from build123d import *

# Parameters (mm, degrees)
SKETCH_1_W               = 25
SKETCH_1_H               = 15
EXTRUDE_1_DEPTH          = 22
FILLET_4_R               = 2
CUT_EXTRUDE_3_DEPTH      = 27.391286441
CUT_EXTRUDE_3_DEPTH_BACK = 27.391286441
CUT_EXTRUDE_4_DEPTH      = 27.391286441
CUT_EXTRUDE_4_DEPTH_BACK = 27.391286441
SKETCH_3_R               = 1
CUT_EXTRUDE_5_DEPTH      = 30.41513216
CUT_EXTRUDE_5_DEPTH_BACK = 30.41513216
SKETCH_4_W               = 13
SKETCH_4_H               = 15
SKETCH_5_W               = 15
SKETCH_5_H               = 7
CUT_EXTRUDE_6_DEPTH      = 35.135758377
FILLET_5_R               = 1


with BuildPart() as part:
    # 草图1 → 凸台-拉伸1 (new body)
    with BuildSketch(Plane.XY):
        Rectangle(SKETCH_1_W, SKETCH_1_H)
    extrude(amount=EXTRUDE_1_DEPTH)

    # 圆角4
    fillet_4_edges = [part.edges().sort_by_distance(p)[0] for p in [
        (12.5, -7.5, 11),
        (-12.5, -7.5, 11),
        (-12.5, 7.5, 11),
        (12.5, 7.5, 11),
    ]]
    fillet(fillet_4_edges, radius=FILLET_4_R)

    # 草图2 → 切除-拉伸3 (cut, two sides: drawn at the far end of the back side and taken through both)
    with BuildSketch(Plane.XY.offset(22).offset(-CUT_EXTRUDE_3_DEPTH_BACK)):
        with BuildLine():
            Line((-10.5, 0.062323454), (-10.5, -0.062323454))
            ThreePointArc((-10.5, -0.062323454), (-10.125727394, -0.842365266), (-9.283069542, -1.038510514))
            Line((-9.283069542, -1.038510514), (-9.002613999, -0.97618706))
            ThreePointArc((-9.002613999, -0.97618706), (-8.219544457, 0), (-9.002613999, 0.97618706))
            Line((-9.002613999, 0.97618706), (-9.283069542, 1.038510514))
            ThreePointArc((-9.283069542, 1.038510514), (-10.125727394, 0.842365266), (-10.5, 0.062323454))
        make_face()
        with BuildLine():
            Line((0.216930458, 1.072600597), (8.997386001, 3.02381294))
            ThreePointArc((8.997386001, 3.02381294), (9.774484481, 4.109116772), (8.780455543, 5))
            Line((8.780455543, 5), (-8.780455543, 5))
            ThreePointArc((-8.780455543, 5), (-9.774484481, 4.109116772), (-8.997386001, 3.02381294))
            Line((-8.997386001, 3.02381294), (-0.216930458, 1.072600597))
            ThreePointArc((-0.216930458, 1.072600597), (0, 1.048787657), (0.216930458, 1.072600597))
        make_face()
        with BuildLine():
            Line((9.283069542, 1.038510514), (9.002613999, 0.97618706))
            ThreePointArc((9.002613999, 0.97618706), (8.219544457, 0), (9.002613999, -0.97618706))
            Line((9.002613999, -0.97618706), (9.283069542, -1.038510514))
            ThreePointArc((9.283069542, -1.038510514), (10.125727394, -0.842365266), (10.5, -0.062323454))
            Line((10.5, -0.062323454), (10.5, 0.062323454))
            ThreePointArc((10.5, 0.062323454), (10.125727394, 0.842365266), (9.283069542, 1.038510514))
        make_face()
        with BuildLine():
            Line((8.780455543, -5), (-8.780455543, -5))
            ThreePointArc((-8.780455543, -5), (-9.774484481, -4.109116772), (-8.997386001, -3.02381294))
            Line((-8.997386001, -3.02381294), (-0.216930458, -1.072600597))
            ThreePointArc((-0.216930458, -1.072600597), (0, -1.048787657), (0.216930458, -1.072600597))
            Line((0.216930458, -1.072600597), (8.997386001, -3.02381294))
            ThreePointArc((8.997386001, -3.02381294), (9.774484481, -4.109116772), (8.780455543, -5))
        make_face()
    extrude(amount=CUT_EXTRUDE_3_DEPTH + CUT_EXTRUDE_3_DEPTH_BACK, mode=Mode.SUBTRACT)

    # 草图3 → 切除-拉伸4 (cut, two sides: drawn at the far end of the back side and taken through both)
    with BuildSketch(Plane.XY.offset(22).offset(-CUT_EXTRUDE_4_DEPTH_BACK)):
        with Locations((-10.5, 5.5)):
            Circle(SKETCH_3_R)
        with Locations(Location((10.5, 5.5, 0), (0, 0, 180))):
            Circle(SKETCH_3_R)
        with Locations((10.5, -5.5)):
            Circle(SKETCH_3_R)
        with Locations(Location((-10.5, -5.5, 0), (0, 0, 180))):
            Circle(SKETCH_3_R)
    extrude(amount=CUT_EXTRUDE_4_DEPTH + CUT_EXTRUDE_4_DEPTH_BACK, mode=Mode.SUBTRACT)

    # 草图4 → 切除-拉伸5 (cut, two sides: drawn at the far end of the back side and taken through both)
    with BuildSketch(Plane(origin=(0, 7.5, 0), x_dir=(1, 0, 0), z_dir=(0, 1, 0)).offset(-CUT_EXTRUDE_5_DEPTH_BACK)):
        with Locations((0, -11)):
            Rectangle(SKETCH_4_W, SKETCH_4_H)
    extrude(amount=CUT_EXTRUDE_5_DEPTH + CUT_EXTRUDE_5_DEPTH_BACK, mode=Mode.SUBTRACT)

    # 草图5 → 切除-拉伸6 (cut, through all)
    with BuildSketch(Plane.ZY.offset(12.5)):
        with Locations((11, 0)):
            Rectangle(SKETCH_5_W, SKETCH_5_H)
    extrude(amount=-CUT_EXTRUDE_6_DEPTH, mode=Mode.SUBTRACT)

    # 圆角5
    fillet_5_edges = [part.edges().sort_by_distance(p)[0] for p in [
        (-6.5, 5, 11),
        (-6.5, 7.5, 11),
        (-6.5, -5, 11),
        (-6.5, -7.5, 11),
        (6.5, 7.5, 11),
        (6.5, 5, 11),
        (6.5, -5, 11),
        (6.5, -7.5, 11),
        (9.646480946, 3.5, 11),
        (-9.646480946, -3.5, 11),
        (9.646480946, -3.5, 11),
        (12.5, -3.5, 11),
        (-9.646480946, 3.5, 11),
        (12.5, 3.5, 11),
        (-12.5, 3.5, 11),
        (-12.5, -3.5, 11),
    ]]
    fillet(fillet_5_edges, radius=FILLET_5_R)


solid = part.part
Build history of the part. All positions in model axes, mm. A direction names the side the tool comes from. Round coordinates to 2 decimals unless told otherwise and drop trailing zeros. Loops run counter-clockwise (first coordinate to the right, second up) from the corner with the lowest first, then second, coordinate; pieces in that order, holes last. Notation, with made-up numbers: (64.5, -18) -> (103.5, -18) arc R36 ccw to (103.5, 21) -> close; hole circle Ø2 at (60, 78). An arc over 180 degrees is marked (long way). One line per item, written item: value. Start each with the question number.
Q1. Cut at D-D on x = 4.5. List the corners of the cut face in (y, z).
Q2. Cut at C-C on x = -5.5. List the corners of the cut face in (y, z), plus the area to 3 significant figures.
Q3. Cut at A-A on y = 1.5. List the corners of the cut face in (x, z).
Q4. Two-plate mould, pull along X, no slides. Class faces 1 (the face through (12.199, 3.785, 11.105)), 2 (the face through (-11.93, 6.9, 11.15)), 3 (the face through (6.801, 7.215, 11.105)): released by +X, released by -X, zero draft, split by the parting line, or undercut.
Q5. Probe line 1 along Z through (x, y) = (3, -6.5); line 2 along Y through (x, z) = (10.5, 4.75); line 3 along Y through (x, z) = (7.75, 20). List the from-to ranges inside material, lowest first.
Q6. 3-axis set-ups, long thin cutter, end or side, ignore diameter. For faces 4 (the face through (-12.215, -3.801, 11.105)), 5 (the face through (-4.669, 2.062, 1.726)), 6 (the face through (-6.801, 5.285, 10.895)): which of +Z, -Z, +X, -X, +Y, -Y reach the whole face in a straight line?
Q7. Drop flat-ended pins along their axis: pin 1 Ø0.6 at (x, z) = (-11, 12.5) entering from +Y; pin 2 Ø0.6 at (y, z) = (6.5, 9.5) entering from +X. Give the stop position or say it passes through.
Q8. Cut at B-B on z = 4. Count the separate pieces of the cut face and the enclosed holes in it, plus the area to 3 significant figures.
Computed:
1. outline: (-7.5, 0) -> (-5, 0) -> (-5, 3.5) -> (-7.5, 3.5) -> close; (-7.5, 18.5) -> (-5, 18.5) -> (-5, 22) -> (-7.5, 22) -> close; (-2.02, 0) -> (2.02, 0) -> (2.02, 3.5) -> (-2.02, 3.5) -> close; (-2.02, 18.5) -> (2.02, 18.5) -> (2.02, 22) -> (-2.02, 22) -> close; (5, 0) -> (7.5, 0) -> (7.5, 3.5) -> (5, 3.5) -> close; (5, 18.5) -> (7.5, 18.5) -> (7.5, 22) -> (5, 22) -> close
2. outline: (-7.5, 0) -> (-5, 0) -> (-5, 3.5) -> (-7.5, 3.5) -> close; (-7.5, 18.5) -> (-5, 18.5) -> (-5, 22) -> (-7.5, 22) -> close; (-2.25, 0) -> (2.25, 0) -> (2.25, 3.5) -> (-2.25, 3.5) -> close; (-2.25, 18.5) -> (2.25, 18.5) -> (2.25, 22) -> (-2.25, 22) -> close; (5, 0) -> (7.5, 0) -> (7.5, 3.5) -> (5, 3.5) -> close; (5, 18.5) -> (7.5, 18.5) -> (7.5, 22) -> (5, 22) -> close
2. area: 66.5 mm²
3. outline: (-12.5, 0) -> (-2.14, 0) -> (-2.14, 3.5) -> (-12.5, 3.5) -> close; (-12.5, 18.5) -> (-2.14, 18.5) -> (-2.14, 22) -> (-12.5, 22) -> close; (2.14, 0) -> (12.5, 0) -> (12.5, 3.5) -> (2.14, 3.5) -> close; (2.14, 18.5) -> (12.5, 18.5) -> (12.5, 22) -> (2.14, 22) -> close
4. face 1: released by +X
4. face 2: released by -X
4. face 3: undercut
5. line 1: 0 to 3.5, 18.5 to 22
5. line 2: -7.5 to -6.5, -4.5 to -3.52, 3.52 to 4.5, 6.5 to 7.5
5. line 3: -7.5 to -5, -2.75 to 2.75, 5 to 7.5
6. face 4: -X
6. face 5: +Z, -Z
6. face 6: none
7. pin 1: y = 7.49
7. pin 2: x = 12.37
8. separate pieces: 4
8. enclosed holes: 4
8. area: 57.9 mm²
